Job drawing, mm, ordinate dimensions from the low corner. One solid piece. A direction names the side the tool comes from. Round coordinates to 2 decimals unless told otherwise and drop trailing zeros. Write each loop counter-clockwise with the first axis right and the second up, starting at its lowest first coordinate (ties: lowest second). Pieces come first, ordered by that corner, then holes. Notation, with made-up numbers: (-9, 32) -> (24, 32) arc R28 cw to (24, 58) -> close; hole circle Ø4 at (-8.5, -19.5). An arc over 180 degrees is marked (long way). Use CSV: the item, a comma, the result in double quotes. Start each with the question number.
(1) Saw through at B-B (y = 16). Give the cut face in (x, z) (3 decimals), plus the area to 3 significant figures.
(2) Saw through at A-A (z = 7.5). Give the cut face in (x, y) (3 decimals).
(3) Probe line 1 (X direction, y = 16.5, z = 8.5); line 2 (Y direction, x = 25, z = 2); line 3 (X direction, y = 9.5, z = 11.25) (3 decimals). List the from-to ranges inside material, lowest first. Write a range as [from, to].
(4) Which spindle directions (+Z, -Z, +X, -X, +Y, -Y) get a long thin tool onto all of the face, cutting with end or side? Do the marked faces 1 and 2. Say none if no direction does.
(5) Two-plate mould, pull along Y, no slides. Class the marked faces 3, 4 and 5: released by +Y, released by -Y, zero draft, split by the parting line, or undercut.
(6) Drop flat-ended pins along their axis: pin 1 (0.6 mm diameter, centred on x = 3.5, z = 11.5, fed in from +Y) (3 decimals); pin 2 (10 mm diameter, centred on x = 16, y = 38.5, fed in from +Z); pin 3 (0.6 mm diameter, centred on y = 13, z = 11.5, fed in from +X) (3 decimals). Give the stop position or say it passes through.
(7) Saw through at C-C (z = 2.5). Give the cut face in (x, y), plus the area to 3 significant figures.
(8) Saw through at D-D (x = 25). Give the cut face in (y, z) (3 decimals), plus the area to 3 significant figures.
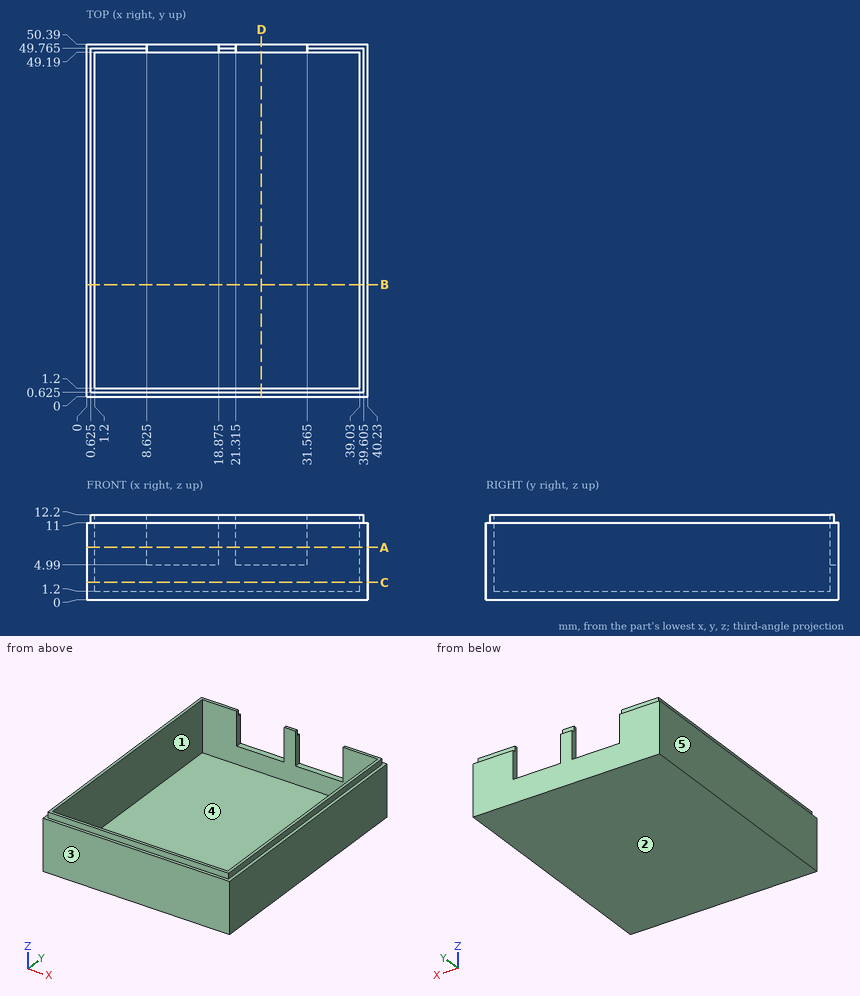
Answers:
1,outline,"(0, 0) -> (40.23, 0) -> (40.23, 11) -> (39.605, 11) -> (39.605, 12.2) -> (39.03, 12.2) -> (39.03, 1.2) -> (1.2, 1.2) -> (1.2, 12.2) -> (0.625, 12.2) -> (0.625, 11) -> (0, 11) -> close"
1,area,"73.2 mm²"
2,outline,"(0, 0) -> (40.23, 0) -> (40.23, 50.39) -> (31.565, 50.39) -> (31.565, 49.19) -> (39.03, 49.19) -> (39.03, 1.2) -> (1.2, 1.2) -> (1.2, 49.19) -> (8.625, 49.19) -> (8.625, 50.39) -> (0, 50.39) -> close; (18.875, 49.19) -> (21.315, 49.19) -> (21.315, 50.39) -> (18.875, 50.39) -> close"
3,line 1,"x = [0, 1.2], [39.03, 40.23]"
3,line 2,"y = [0, 1.2], [49.19, 50.39]"
3,line 3,"x = [0.625, 1.2], [39.03, 39.605]"
4,face 1,"+Z"
4,face 2,"-Z, +X, -X, +Y, -Y"
5,face 3,"released by -Y"
5,face 4,"undercut"
5,face 5,"zero draft"
6,pin 1,"stops at y = 49.765"
6,pin 2,"stops at z = 1.2"
6,pin 3,"stops at x = 39.605"
7,outline,"(0, 0) -> (40.23, 0) -> (40.23, 50.39) -> (0, 50.39) -> close; hole (1.2, 1.2) -> (39.03, 1.2) -> (39.03, 49.19) -> (1.2, 49.19) -> close"
7,area,"212 mm²"
8,outline,"(0, 0) -> (50.39, 0) -> (50.39, 4.99) -> (49.19, 4.99) -> (49.19, 1.2) -> (1.2, 1.2) -> (1.2, 12.2) -> (0.625, 12.2) -> (0.625, 11) -> (0, 11) -> close"
8,area,"77.5 mm²"
